Design review of the part built by this model. Coordinates are the model's own, in mm. A direction names the side the tool comes from. Give positions to 0.01 mm unless a question says otherwise; leave off trailing zeros. Loops run counter-clockwise (first coordinate to the right, second up) from the corner with the lowest first, then second, coordinate; pieces in that order, holes last. Notation, with made-up numbers: (-31, 41.25) - (-7, 41.25) arc R21 cw to (-7, 64.25) - close; hole circle Ø5 at (-3.75, 80.5). An arc over 180 degrees is marked (long way). Write each question's results on one line, items separated by ' | '.
```python
from build123d import *


with BuildPart() as part:
    # Szkic1 → Obrót1 (revolve)
    with BuildSketch(Plane.XY, mode=Mode.PRIVATE) as obr_t1_sk:
        with BuildLine():
            Line((-31.319935083, 63.856960175), (-25.319935083, 63.856960175))
            Line((-25.319935083, 63.856960175), (-25.319935083, 55.856960175))
            ThreePointArc((-25.319935083, 55.856960175), (-8.395162691, 35.250864878), (0, 9.941176471))
            Line((0, 9.941176471), (0, 5))
            Line((0, 5), (1, 5))
            Line((1, 5), (1, 10.0093516))
            ThreePointArc((1, 10.0093516), (-7.390646301, 35.49911912), (-24.319935083, 56.320511361))
            Line((-24.319935083, 56.320511361), (-24.319935083, 64.856960175))
            Line((-24.319935083, 64.856960175), (-31.319935083, 64.856960175))
            Line((-31.319935083, 64.856960175), (-31.319935083, 63.856960175))
        make_face()
    revolve(obr_t1_sk.sketch.rotate(Axis((-67.855420072, 0, 0), (1, 0, 0)), 90), axis=Axis((-67.855420072, 0, 0), (1, 0, 0)))


solid = part.part
```
Item 1: Draft analysis for pull direction Z (two halves, no side actions). For faces 4 (the face through (1, 2, 5)), 5 (the face through (-27.869, -19.481, 61.862)), 6 (the face through (-28.28, -19.18, 60.91)), 7 (the face through (0, -5, 2)), state which applies: +Z half, -Z half, draft (parallel to the pull), parting line (faces both ways), or undercut.
Output values:
face 4: draft | face 5: parting line | face 6: undercut | face 7: undercut
Item 2: Clearance check with flat-ended pins moving along their axes: P1, Ø4, axis at x = -24.5, y = 32.5, coming from the +Z side; P2, Ø1, axis at y = -3.5, z = 23.5, coming from the +X side; P3, Ø3, axis at x = -26, z = -40.5, coming from the -Y side. State where each tip first meets the part, or that it passes through.
Output values:
P1: stops at z = 57.24 | P2: stops at x = -2.07 | P3: stops at y = -51.82
Item 3: We need section D-D on z = -50. Give the boundary of the cut face in (x, y).
Output values:
outline: (-31.32, -41.31) - (-24.32, -41.31) - (-24.32, -25.92) arc R54.55 ccw to (-24.32, 25.92) - (-24.32, 41.31) - (-31.32, 41.31) - (-31.32, 39.72) - (-25.32, 39.72) - (-25.32, 24.9) arc R53.19 cw to (-25.32, -24.9) - (-25.32, -39.72) - (-31.32, -39.72) - close
Item 4: Tool access review of faces 1 (the face through (-31.32, 43, 48)), 2 (the face through (-24.32, -53, 20)), 3 (the face through (-25.32, 56.5, -0.3)): name each direction out of +Z, -Z, +X, -X, +Y, -Y from which nothing blocks a thin tool from reaching the whole face with its end or side.
Output values:
face 1: +Z, -Z, -X, +Y, -Y | face 2: +X | face 3: -X
Item 5: We need section C-C on y = -20.5. Give the boundary of the cut face in (x, z).
Output values:
outline: (-31.32, -61.53) - (-24.32, -61.53) - (-24.32, -52.46) arc R71.1 ccw to (-24.32, 52.46) - (-24.32, 61.53) - (-31.32, 61.53) - (-31.32, 60.48) - (-25.32, 60.48) - (-25.32, 51.96) arc R70.06 cw to (-25.32, -51.96) - (-25.32, -60.48) - (-31.32, -60.48) - close
Item 6: We need section A-A on y = 0. Give the boundary of the cut face in (x, z).
Output values:
outline: (-31.32, -64.86) - (-24.32, -64.86) - (-24.32, -56.32) arc R74 ccw to (1, -10.01) - (1, -5) - (0, -5) - (0, -9.94) arc R73 cw to (-25.32, -55.86) - (-25.32, -63.86) - (-31.32, -63.86) - close; (-31.32, 63.86) - (-25.32, 63.86) - (-25.32, 55.86) arc R73 cw to (0, 9.94) - (0, 5) - (1, 5) - (1, 10.01) arc R74 ccw to (-24.32, 56.32) - (-24.32, 64.86) - (-31.32, 64.86) - close
Item 7: Wall thickness on probe 1 along Y at (x, z) = (-30, 0.5) (3 decimals); probe 2 along Z at (x, y) = (-10.5, 25.5); probe 3 along X at (y, z) = (-3, -9): over which ranges is each line inside the solid? List them lowest first.
Output values:
probe 1: y = -64.855 to -63.855, 63.855 to 64.855 | probe 2: z = -31.69 to -29.28, 29.28 to 31.69 | probe 3: x = 0 to 1
